Geometry: see drawing. Coordinates: mm, zero at the bounding-box minimum. Coordinates: 2 decimals unless noted, no trailing zeros. Loops run counter-clockwise (first coordinate to the right, second up) from the corner with the lowest first, then second, coordinate; pieces in that order, holes last. Notation, with made-up numbers: (12.25, -7) -> (19.25, -7) arc R27 ccw to (19.25, 29) -> close; hole circle Ø9 at (-20.75, 42). An arc over 180 degrees is marked (long way). One line per item, written item: value. Start each with the question number.
Item 1: Contact query for flat-ended pins moving along their axis: pin 1 Ø1 at (x, z) = (19.5, 1.5) entering from +Y; pin 2 Ø1 at (x, z) = (21.5, 2.5) entering from -Y. Output: stop coordinate, or through.
Item 2: Section query A-A on y = 13.5. Return loops of the section in (x, z), then the cut area to 3 significant figures.
Item 3: Section query C-C on z = 1.45. Return loops of the section in (x, y), then the cut area to 3 significant figures.
Item 4: Ray query, probe 1 along Y at (x, z) = (13.5, 0.75); probe 2 along X at (y, z) = (13.25, 1); probe 3 along X at (y, z) = (12.75, 1). Return the intervals inside material, ascending. Write a range as from..to.
Item 5: Mould query, pull axis X, two halves, no side actions, for the marked faces 1, 2 and 3. Classes: +X half, -X half, draft (parallel to the pull), parting line (faces both ways), or undercut.
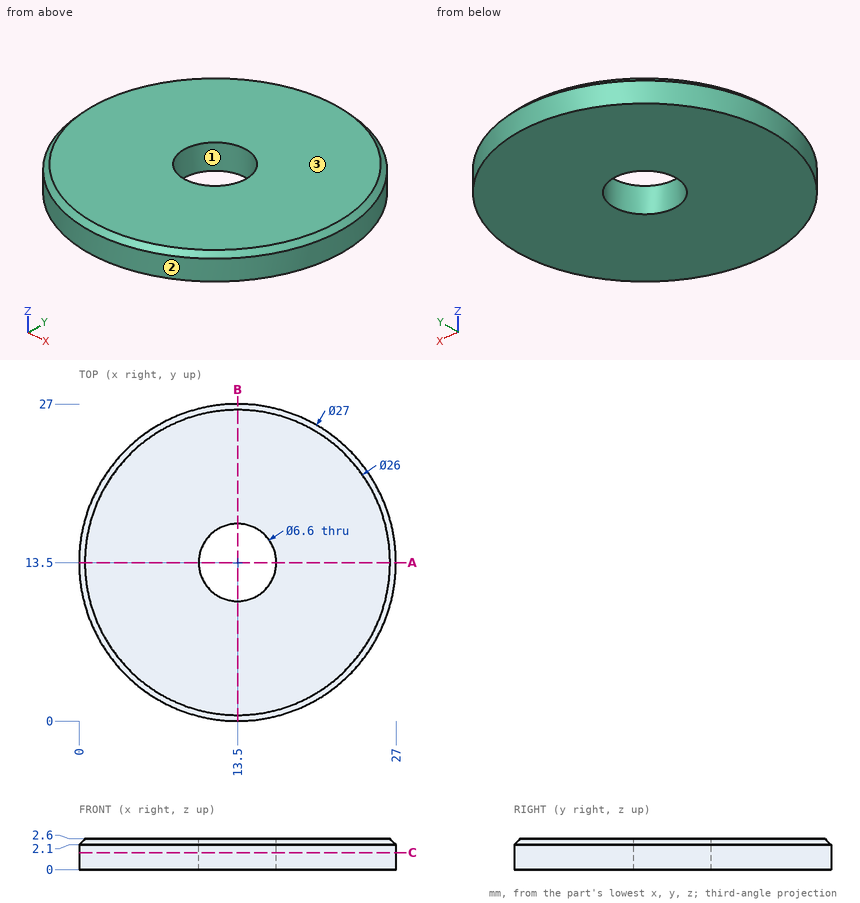
Reply:
1. pin 1: stops at y = 25.83
1. pin 2: stops at y = 2.41
2. outline: (0, 0) -> (10.2, 0) -> (10.2, 2.6) -> (0.5, 2.6) -> (0, 2.1) -> close; (16.8, 0) -> (27, 0) -> (27, 2.1) -> (26.5, 2.6) -> (16.8, 2.6) -> close
2. area: 52.8 mm²
3. outline: circle Ø27 at (13.5, 13.5); hole circle Ø6.6 at (13.5, 13.5)
3. area: 538 mm²
4. probe 1: y = 0..10.2, 16.8..27
4. probe 2: x = 0..10.21, 16.79..27
4. probe 3: x = 0.02..10.29, 16.71..26.98
5. face 1: undercut
5. face 2: parting line
5. face 3: draft
